from build123d import *

# Parameters (mm, degrees)
F0_W     = 50
F0_H     = 10
F1_DEPTH = 5
F2_R     = 1.5
F3_DEPTH = 5.001
F5_R     = 4.99999
F4_R     = 2.91
F4_R_2   = 2.935
F4_R_3   = 2.96
F4_R_4   = 2.985
F4_R_5   = 3.01
F6_DEPTH = 3.6


# Not quite as in the source:
# - a fillet or chamfer is up to 0.001 mm smaller than in the source, because OpenCascade refuses the exact size


with BuildPart() as f1:
    # F0 (on Top) → F1 (new body)
    with BuildSketch(Plane.XY):
        with Locations((25, 5)):
            Rectangle(F0_W, F0_H)
    extrude(amount=F1_DEPTH)

    # F2 (on face) → F3 (cut, through all)
    with BuildSketch(Plane(origin=(0, 0, 0), x_dir=(1, 0, 0), z_dir=(0, 0, -1))):
        with Locations((5, -5)):
            Circle(F2_R)
        with Locations((15, -5)):
            Circle(F2_R)
        with Locations((25, -5)):
            Circle(F2_R)
        with Locations((35, -5)):
            Circle(F2_R)
        with Locations((45, -5)):
            Circle(F2_R)
    extrude(amount=-F3_DEPTH, mode=Mode.SUBTRACT)

    # F5 (radius 5 in the source; OpenCascade refuses exactly that, so slightly less here)
    f5_edges = [f1.edges().sort_by_distance(p)[0] for p in [
        (0, 0, 2.5),
        (0, 10, 2.5),
        (50, 0, 2.5),
        (50, 10, 2.5),
    ]]
    fillet(f5_edges, radius=F5_R)

    # F4 (on face) → F6 (cut)
    with BuildSketch(Plane.XY.offset(5)):
        with Locations((5, 5)):
            Circle(F4_R)
        with Locations((15, 5)):
            Circle(F4_R_2)
        with Locations((25, 5)):
            Circle(F4_R_3)
        with Locations((35, 5)):
            Circle(F4_R_4)
        with Locations((45, 5)):
            Circle(F4_R_5)
    extrude(amount=-F6_DEPTH, mode=Mode.SUBTRACT)


solid = f1.part
Geometry: final body of the model. Coordinates: model frame, mm. A direction names the side the tool comes from. Coordinates: 2 decimals unless noted, no trailing zeros. Order: outer loops, then holes, each group sorted by start corner. A loop starts at its lowest first (then second) coordinate and runs counter-clockwise, first axis right, second up.
(1) First-contact query: pin 1 (3 mm diameter, centred on x = 6, y = 3.5, fed in from +Z); pin 2 (1 mm diameter, centred on y = 4, z = 2.5, fed in from +X); pin 3 (3 mm diameter, centred on x = 35.5, y = 5, fed in from +Z); pin 4 (1.5 mm diameter, centred on y = 7.5, z = 4, fed in from -X). Flat tips, straight axial feed; report the tip coordinate or a pass-through.
(2) Draft query along Y for faces 3 (the face through (37.847, 5.897, 3.225)), 4 (the face through (25, 0, 2)), 5 (the face through (25, 7, 0)). Return one class per face: pulls with the +Y half, pulls with the -Y half, needs draft (parallel to the pull), parting line crosses it, or undercut.
(3) Section query A-A (x = 25). Return the cut outline in (y, z), plus the area to 3 significant figures.
(4) Access query for faces 1 (the face through (26.3, 3.7, 1.4)), 2 (the face through (5.806, 3.735, 0.69)). Directions: +Z, -Z, +X, -X, +Y, -Y. A direction counts if a zero-diameter tool reaches every point of the face in a straight line with its end or side. Return the directions, or none.
(5) Section query B-B (z = 4.3). State how many separate pieces and enclosed holes the cut face has, plus the area to 3 significant figures.
(6) Material intervals for probe 1 along X at (y, z) = (5, 1); probe 2 along X at (y, z) = (4.25, 1.8); probe 3 along Y at (x, z) = (25, 3.3), sorted ascending.
(7) Section query D-D (y = 7.25). Return the cut outline in (x, z).
(8) Section query C-C (x = 15). Return the cut outline in (y, z) (3 decimals), plus the area to 3 significant figures.
Solution:
1. pin 1: stops at z = 5
1. pin 2: stops at x = 49.97
1. pin 3: stops at z = 1.4
1. pin 4: stops at x = 0.32
2. face 3: undercut
2. face 4: pulls with the -Y half
2. face 5: needs draft
3. outline: (0, 0) - (3.5, 0) - (3.5, 1.4) - (2.04, 1.4) - (2.04, 5) - (0, 5) - close; (6.5, 0) - (10, 0) - (10, 5) - (7.96, 5) - (7.96, 1.4) - (6.5, 1.4) - close
3. area: 24.5 mm2
4. face 1: +Z
4. face 2: +Z, -Z
5. separate pieces: 1
5. enclosed holes: 5
5. area: 341 mm2
6. probe 1: x = 0 to 3.5, 6.5 to 13.5, 16.5 to 23.5, 26.5 to 33.5, 36.5 to 43.5, 46.5 to 50
6. probe 2: x = 0.06 to 2.19, 7.81 to 12.16, 17.84 to 22.14, 27.86 to 32.11, 37.89 to 42.08, 47.92 to 49.94
6. probe 3: y = 0 to 2.04, 7.96 to 10
7. outline: (0.53, 0) - (49.47, 0) - (49.47, 5) - (47, 5) - (47, 1.4) - (43, 1.4) - (43, 5) - (36.96, 5) - (36.96, 1.4) - (33.04, 1.4) - (33.04, 5) - (26.92, 5) - (26.92, 1.4) - (23.08, 1.4) - (23.08, 5) - (16.88, 5) - (16.88, 1.4) - (13.12, 1.4) - (13.12, 5) - (6.85, 5) - (6.85, 1.4) - (3.15, 1.4) - (3.15, 5) - (0.53, 5) - close
8. outline: (0, 0) - (3.5, 0) - (3.5, 1.4) - (2.065, 1.4) - (2.065, 5) - (0, 5) - close; (6.5, 0) - (10, 0) - (10, 5) - (7.935, 5) - (7.935, 1.4) - (6.5, 1.4) - close
8. area: 24.7 mm2
